The model under review builds one solid part; all positions refer to its coordinate system, in mm. A direction names the side the tool comes from. Round coordinates to 2 decimals unless told otherwise and drop trailing zeros. Write each loop counter-clockwise with the first axis right and the second up, starting at its lowest first coordinate (ties: lowest second). Pieces come first, ordered by that corner, then holes. Notation, with made-up numbers: (-30, 26) - (-3, 26) arc R10 cw to (-3, 39) - close; hole circle Ø4 at (32, 36.5). An arc over 180 degrees is marked (long way). Return JSON: item names as keys, results as strings.
from build123d import *

# Parameters (mm, degrees)
BOSS_EXTRUDE1_DEPTH = 100
SKETCH2_W           = 5
SKETCH2_H           = 55
CUT_EXTRUDE2_DEPTH  = 5
SKETCH3_W           = 5
SKETCH3_H           = 55
CUT_EXTRUDE3_DEPTH  = 5
SKETCH4_W           = 15
SKETCH4_H           = 5
CUT_EXTRUDE4_DEPTH  = 5
SKETCH5_W           = 15
SKETCH5_H           = 5
CUT_EXTRUDE5_DEPTH  = 5
SKETCH6_R           = 6
CUT_EXTRUDE6_DEPTH  = 10
SKETCH7_W           = 5
SKETCH7_H           = 90
BOSS_EXTRUDE2_DEPTH = 55
SKETCH8_R           = 6
CUT_EXTRUDE7_DEPTH  = 80
SKETCH9_W           = 5
SKETCH9_H           = 25
CUT_EXTRUDE8_DEPTH  = 100
SKETCH10_W          = 5
SKETCH10_H          = 5
CUT_EXTRUDE9_DEPTH  = 5
SKETCH11_W          = 5
SKETCH11_H          = 5
CUT_EXTRUDE10_DEPTH = 5
SKETCH12_W          = 50
SKETCH12_H          = 5
BOSS_EXTRUDE3_DEPTH = 55


with BuildPart() as part:
    # Sketch1 → Boss-Extrude1 (new body)
    with BuildSketch(Plane.XY):
        Polygon((0, 0), (-65, 0), (-65, -55), (-70, -55), (-70, 0), (-70, 30), (-65, 30), (-65, 5), (0, 5), align=None)
    extrude(amount=BOSS_EXTRUDE1_DEPTH)

    # Sketch2 → Cut-Extrude2 (cut)
    with BuildSketch(Plane.XY.offset(100)):
        with Locations((-67.5, -27.5)):
            Rectangle(SKETCH2_W, SKETCH2_H)
    extrude(amount=-CUT_EXTRUDE2_DEPTH, mode=Mode.SUBTRACT)

    # Sketch3 → Cut-Extrude3 (cut)
    with BuildSketch(Plane(origin=(0, 0, 0), x_dir=(-1, 0, 0), z_dir=(0, 0, -1))):
        with Locations((67.5, -27.5)):
            Rectangle(SKETCH3_W, SKETCH3_H)
    extrude(amount=-CUT_EXTRUDE3_DEPTH, mode=Mode.SUBTRACT)

    # Sketch4 → Cut-Extrude4 (cut)
    with BuildSketch(Plane.XY.offset(100)):
        with Locations((-57.5, 2.5)):
            Rectangle(SKETCH4_W, SKETCH4_H)
    extrude(amount=-CUT_EXTRUDE4_DEPTH, mode=Mode.SUBTRACT)

    # Sketch5 → Cut-Extrude5 (cut)
    with BuildSketch(Plane(origin=(0, 0, 0), x_dir=(-1, 0, 0), z_dir=(0, 0, -1))):
        with Locations((57.5, 2.5)):
            Rectangle(SKETCH5_W, SKETCH5_H)
    extrude(amount=-CUT_EXTRUDE5_DEPTH, mode=Mode.SUBTRACT)

    # Sketch6 → Cut-Extrude6 (cut)
    with BuildSketch(Plane(origin=(0, 5, 0), x_dir=(1, 0, 0), z_dir=(0, 1, 0))):
        with Locations(Location((-50, -65, 0), (0, 0, 180))):
            Circle(SKETCH6_R)
    extrude(amount=-CUT_EXTRUDE6_DEPTH, mode=Mode.SUBTRACT)

    # Sketch7 → Boss-Extrude2 (add)
    with BuildSketch(Plane.XZ):
        with Locations((-12.5, 50)):
            Rectangle(SKETCH7_W, SKETCH7_H)
    extrude(amount=BOSS_EXTRUDE2_DEPTH)

    # Sketch8 → Cut-Extrude7 (cut)
    with BuildSketch(Plane.ZY.offset(70)):
        with Locations(Location((55, -35, 0), (0, 0, 270))):
            Circle(SKETCH8_R)
    extrude(amount=-CUT_EXTRUDE7_DEPTH, mode=Mode.SUBTRACT)

    # Sketch9 → Cut-Extrude8 (cut)
    with BuildSketch(Plane.XY.offset(100)):
        with Locations((-67.5, 17.5)):
            Rectangle(SKETCH9_W, SKETCH9_H)
    extrude(amount=-CUT_EXTRUDE8_DEPTH, mode=Mode.SUBTRACT)

    # Sketch10 → Cut-Extrude9 (cut)
    with BuildSketch(Plane.XY.offset(100)):
        with Locations((-67.5, 2.5)):
            Rectangle(SKETCH10_W, SKETCH10_H)
    extrude(amount=-CUT_EXTRUDE9_DEPTH, mode=Mode.SUBTRACT)

    # Sketch11 → Cut-Extrude10 (cut)
    with BuildSketch(Plane(origin=(0, 0, 0), x_dir=(-1, 0, 0), z_dir=(0, 0, -1))):
        with Locations((67.5, 2.5)):
            Rectangle(SKETCH11_W, SKETCH11_H)
    extrude(amount=-CUT_EXTRUDE10_DEPTH, mode=Mode.SUBTRACT)

    # Sketch12 → Boss-Extrude3 (add)
    with BuildSketch(Plane.XZ):
        with Locations((-40, 7.5)):
            Rectangle(SKETCH12_W, SKETCH12_H)
        with Locations((-40, 92.5)):
            Rectangle(SKETCH12_W, SKETCH12_H)
    extrude(amount=BOSS_EXTRUDE3_DEPTH)


solid = part.part
(1) Mouldability with a two-part tool opening along X and no side actions: class faces 5 (the flat face through (0, 3, 49)), 6 (the cylindrical face through (-13, -29, 55)), 7 (the flat face through (-40, -27, 90)) as released by +X, released by -X, zero draft, split by the parting line, or undercut.
Filled in:
{"face 5": "released by +X", "face 6": "zero draft", "face 7": "undercut"}
(2) Add section A-A (y = -35). Write out the cut boundary in (x, z).
Filled in:
{"outline": "(-70, 5) - (-10, 5) - (-10, 49) - (-15, 49) - (-15, 10) - (-65, 10) - (-65, 49) - (-70, 49) - close; (-70, 61) - (-65, 61) - (-65, 90) - (-15, 90) - (-15, 61) - (-10, 61) - (-10, 95) - (-70, 95) - close"}
(3) Clearance check with flat-ended pins moving along their axes: pin 1 Ø10 at (x, y) = (-13, -44) entering from -Z; pin 2 Ø25 at (x, y) = (-47.5, -21) entering from +Z; pin 3 Ø5 at (y, z) = (-46, 25.5) entering from +X; pin 4 Ø7 at (x, z) = (-50, 65) entering from -Y. State where each tip first meets the part, or that it passes through.
Filled in:
{"pin 1": "stops at z = 5", "pin 2": "stops at z = 95", "pin 3": "stops at x = -10", "pin 4": "passes through"}
(4) For faces 1 (the flat face through (-10, -27, 49)), 2 (the flat face through (-40, 0, 49)), 3 (the flat face through (-50, 2, 2)), 4 (the flat face through (-50, 2, 98)), list the 3-axis set-ups (+Z, -Z, +X, -X, +Y, -Y) from which the entire face can be reached by the end or side of a thin tool; tool diameter is ignored.
Filled in:
{"face 1": "+Z, -Z, +X, -Y", "face 2": "-Y", "face 3": "-Z, -X, +Y, -Y", "face 4": "+Z, -X, +Y, -Y"}
(5) Wall thickness on line 1 (Z direction, x = -39, y = -42.5); line 2 (X direction, y = -51.5, z = 27); line 3 (Z direction, x = -11.1, y = -35): over which ranges is each line inside the solid? List them lowest first.
Filled in:
{"line 1": "z = 5 to 10, 90 to 95", "line 2": "x = -70 to -65, -15 to -10", "line 3": "z = 5 to 49, 61 to 95"}
(6) Add section B-B (z = 55). Write out the cut boundary in (x, y), plus the area to 3 significant figures.
Filled in:
{"outline": "(-70, -55) - (-65, -55) - (-65, -41) - (-70, -41) - close; (-70, -29) - (-65, -29) - (-65, 0) - (-15, 0) - (-15, -29) - (-10, -29) - (-10, 0) - (0, 0) - (0, 5) - (-70, 5) - close; (-15, -55) - (-10, -55) - (-10, -41) - (-15, -41) - close", "area": "780 mm2"}
(7) Add section D-D (z = 65). Write out the cut boundary in (x, y), plus the area to 3 significant figures.
Filled in:
{"outline": "(-70, -55) - (-65, -55) - (-65, 0) - (-56, 0) - (-56, 5) - (-70, 5) - close; (-44, 0) - (-15, 0) - (-15, -55) - (-10, -55) - (-10, 0) - (0, 0) - (0, 5) - (-44, 5) - close", "area": "840 mm2"}
(8) Add section C-C (y = -21). Write out the cut boundary in (x, z).
Filled in:
{"outline": "(-70, 5) - (-10, 5) - (-10, 95) - (-70, 95) - close; hole (-65, 10) - (-15, 10) - (-15, 90) - (-65, 90) - close"}
